The model under review builds one solid part; all positions refer to its coordinate system, in mm. A direction names the side the tool comes from. Round coordinates to 2 decimals unless told otherwise and drop trailing zeros. Loops run counter-clockwise (first coordinate to the right, second up) from the corner with the lowest first, then second, coordinate; pieces in that order, holes last. Notation, with made-up numbers: (69.5, -29.75) - (126.5, -29.75) arc R26 ccw to (126.5, -8.75) - close; hole circle Ø6 at (25.5, 67.5). An arc over 180 degrees is marked (long way). Answer as CSV lines item,"result".
from build123d import *

# Parameters (mm, degrees)
CYLINDER005_R             = 1.2
CYLINDER005_DEPTH         = 32
CYLINDER005_ROLL_ANGLE    = 90
CYLINDER004_R             = 4
CYLINDER004_DEPTH         = 15
CYLINDER004_ROLL_ANGLE    = 90
CYLINDER003_R             = 25
CYLINDER003_DEPTH         = 15
CYLINDER003_ROLL_ANGLE    = 90
THICKNESS001_T            = -3
FUSION001_PLACEMENT_ANGLE = 180


with BuildPart() as wheelshaft:
    # Cylinder005 → Cylinder005 (new body)
    with BuildSketch(Plane.XY):
        Circle(CYLINDER005_R)
    extrude(amount=CYLINDER005_DEPTH)


with BuildPart() as wheelshaft_1:
    # Cylinder005 roll: moved
    add(wheelshaft.part.rotate(Axis((0, 0, 0), (1, 0, 0)), CYLINDER005_ROLL_ANGLE))


with BuildPart() as wheelshaft_2:
    # Cylinder005 placement: moved
    add(wheelshaft_1.part.moved(Location((0, 40, 0))))


with BuildPart() as shaft_holder_b:
    # Cylinder004 → Cylinder004 (new body)
    with BuildSketch(Plane.XY):
        Circle(CYLINDER004_R)
    extrude(amount=CYLINDER004_DEPTH)


with BuildPart() as shaft_holder_b_1:
    # Cylinder004 roll: moved
    add(shaft_holder_b.part.rotate(Axis((0, 0, 0), (1, 0, 0)), CYLINDER004_ROLL_ANGLE))


with BuildPart() as shaft_holder_b_2:
    # Cylinder004 placement: moved
    add(shaft_holder_b_1.part.moved(Location((0, -23, 0))))


with BuildPart() as wheel_shaft_hollow_b:
    # Cylinder003 → Cylinder003 (new body)
    with BuildSketch(Plane.XY):
        Circle(CYLINDER003_R)
    extrude(amount=CYLINDER003_DEPTH)


with BuildPart() as wheel_shaft_hollow_b_1:
    # Cylinder003 roll: moved
    add(wheel_shaft_hollow_b.part.rotate(Axis((0, 0, 0), (1, 0, 0)), CYLINDER003_ROLL_ANGLE))


with BuildPart() as wheel_shaft_hollow_b_2:
    # Cylinder003 placement: moved
    add(wheel_shaft_hollow_b_1.part.moved(Location((0, -23, 0))))

    # Thickness001
    thickness001_openings = [wheel_shaft_hollow_b_2.faces().sort_by_distance(p)[0] for p in [
        (0, -38, 0),
    ]]
    offset(amount=THICKNESS001_T, openings=thickness001_openings)

    # Fusion001: union shaft_holder_b
    add(shaft_holder_b_2.part)


with BuildPart() as wheel_shaft_hollow_b_3:
    # Fusion001 placement: moved
    add(wheel_shaft_hollow_b_2.part.rotate(Axis((0, 0, 0), (0, 0, 1)), FUSION001_PLACEMENT_ANGLE))

    # Cut001: cut wheelshaft
    add(wheelshaft_2.part, mode=Mode.SUBTRACT)


solid = wheel_shaft_hollow_b_3.part
1. Clearance check with flat-ended pins moving along their axes: pin 1 (6 mm diameter, centred on x = -13, z = 10, fed in from +Y); pin 2 (1.4 mm diameter, centred on x = 0, z = 0, fed in from +Y); pin 3 (4 mm diameter, centred on x = -5.5, y = 27.5, fed in from +Z); pin 4 (2 mm diameter, centred on x = 18, y = 30, fed in from -Z). State where each tip first meets the part, or that it passes through.
Numbers:
pin 1,"stops at y = 26"
pin 2,"passes through"
pin 3,"stops at z = 24.75"
pin 4,"stops at z = -18.33"
2. Tool access review of faces 1 (the face through (4.769, 31.916, -21.477)), 2 (the face through (-1, 38, 1)): name each direction out of +Z, -Z, +X, -X, +Y, -Y from which nothing blocks a thin tool from reaching the whole face with its end or side.
Numbers:
face 1,"+Y"
face 2,"+Z, -Z, +X, -X, +Y"
3. Draft analysis for pull direction Z (two halves, no side actions). For faces 3 (the face through (-1.7, 38, -22.1)), 4 (the face through (-23.846, 30.395, 7.509)), 5 (the face through (0.65, 30.6, 1.01)), 6 (the face through (0.867, 31.916, -3.905)), state which applies: +Z half, -Z half, draft (parallel to the pull), parting line (faces both ways), or undercut.
Numbers:
face 3,"draft"
face 4,"parting line"
face 5,"undercut"
face 6,"undercut"
4. Take a section at A-A (x = 0). State the section outline as (y, z) points, plus the area to 3 significant figures.
Numbers:
outline,"(23, -25) - (38, -25) - (38, -22) - (26, -22) - (26, -4) - (38, -4) - (38, -1.2) - (23, -1.2) - close; (23, 1.2) - (38, 1.2) - (38, 4) - (26, 4) - (26, 22) - (38, 22) - (38, 25) - (23, 25) - close"
area,"282 mm²"
5. Take a section at D-D (x = 19). State the section outline as (y, z) points, plus the area to 3 significant figures.
Numbers:
outline,"(23, -16.25) - (38, -16.25) - (38, -11.09) - (26, -11.09) - (26, 11.09) - (38, 11.09) - (38, 16.25) - (23, 16.25) - close"
area,"221 mm²"
6. Take a section at C-C (z = 0). State the section outline as (x, y) points, plus the area to 3 significant figures.
Numbers:
outline,"(-25, 23) - (-1.2, 23) - (-1.2, 38) - (-4, 38) - (-4, 26) - (-22, 26) - (-22, 38) - (-25, 38) - close; (1.2, 23) - (25, 23) - (25, 38) - (22, 38) - (22, 26) - (4, 26) - (4, 38) - (1.2, 38) - close"
area,"282 mm²"
7. Take a section at B-B (y = 32.25). State the section outline as (x, z) points, plus the area to 3 significant figures.
Numbers:
outline,"circle Ø50 at (0, 0); circle Ø8 at (0, 0); hole circle Ø44 at (0, 0); hole circle Ø2.4 at (0, 0)"
area,"489 mm²"
8. Wall thickness on probe 1 along Z at (x, y) = (0, 29.5); probe 2 along X at (y, z) = (35, 2.5); probe 3 along Y at (x, z) = (3.5, -20): over which ranges is each line inside the solid? List them lowest first.
Numbers:
probe 1,"z = -25 to -22, -4 to -1.2, 1.2 to 4, 22 to 25"
probe 2,"x = -24.87 to -21.86, -3.12 to 3.12, 21.86 to 24.87"
probe 3,"y = 23 to 26"
